Source: CAD feature listing. Evaluate the final solid. Frame: model axes, mm. A direction names the side the tool comes from. Round coordinates to 2 decimals unless told otherwise and drop trailing zeros. Order: outer loops, then holes, each group sorted by start corner. A loop starts at its lowest first (then second) coordinate and runs counter-clockwise, first axis right, second up. Notation, with made-up numbers: (68.25, -22) - (96.25, -22) arc R31 ccw to (96.25, 2) - close; hole circle Ø11 at (57, 14). An arc over 180 degrees is marked (long way). Return JSON: item names as keys, results as strings. Group by question number.
1) Section C-C, the plane y = 17.5. Return loops of the section in (x, z).
2) Ray query, line 1 (Y direction, x = 24.5, z = 0.05); line 2 (Y direction, x = 24.5, z = 9); line 3 (X direction, y = 18.5, z = 1). Return the intervals inside material, ascending. Write a range as from..to.
3) Section A-A, the plane x = -24.5. Return loops of the section in (y, z).
4) Section D-D, the plane x = 21.5. Return loops of the section in (y, z), plus the area to 4 significant figures.
5) Mould query, pull axis Y, two halves, no side actions, for faces 1 (the flat face through (28, 22.5, 5)), 2 (the flat face through (20, 18, 5)), 3 (the flat face through (27, 12.5, 5)). Classes: pulls with the +Y half, pulls with the -Y half, needs draft (parallel to the pull), parting line crosses it, or undercut.
6) Access query for faces 4 (the flat face through (35, 17, 5)), 5 (the flat face through (31, 18, 0.1)). Directions: +Z, -Z, +X, -X, +Y, -Y. A direction counts if a zero-diameter tool reaches every point of the face in a straight line with its end or side. Return the directions, or none.
7) Contact query for flat-ended pins moving along their axis: P1, Ø2.5, axis at x = 24.5, y = 24.5, coming from the -Z side; P2, Ø6.5, axis at x = -24.5, y = 24.5, coming from the +Z side; P3, Ø5, axis at y = 19, z = 7, coming from the -X side. Output: stop coordinate, or through.
Autodesk Inventor part; units mm, degrees
ref_plane "YZ Plane" through (0, 0, 0) normal (1, 0, 0) x (0, 1, 0)
ref_plane "XZ Plane" through (0, 0, 0) normal (0, 1, 0) x (-1, 0, 0)
ref_plane "XY Plane" through (0, 0, 0) normal (0, 0, 1) x (1, 0, 0)
sketch "스케치2" plane through (0, 0, 0) normal (0, 0, 1) x (1, 0, 0)
  line L0 (-27.5, 27.5) -> (27.5, 27.5)
  line L1 (27.5, 27.5) -> (27.5, -27.5)
  line L2 (27.5, -27.5) -> (-27.5, -27.5)
  line L3 (-27.5, -27.5) -> (-27.5, 27.5)
  line L4 (-27.5, 27.5) -> (27.5, -27.5) construction
  line L5 (27.5, 27.5) -> (-27.5, -27.5) construction
  point P0 (0, 0)
  dimension "d0" = 55
  dimension "d1" = 55
extrude "돌출1" add sketch "스케치2" along normal blind 0.1
sketch "스케치3" plane through (0, 0, 0.1) normal (0, 0, 1) x (1, 0, 0)
  line L0 (27.5, -27.5) -> (27.5, 27.5)
  line L1 (27.5, 27.5) -> (-27.5, 27.5)
  circle A0 centre (24.5, 24.5) radius 3
  circle A1 centre (-24.5, 24.5) radius 3
  circle A2 centre (-24.5, -24.5) radius 3
  circle A3 centre (24.5, -24.5) radius 3
  line L2 (-27.5, 27.5) -> (-27.5, -27.5)
  line L3 (-27.5, -27.5) -> (27.5, -27.5)
  circle A4 centre (24.5, 24.5) radius 2
  circle A5 centre (-24.5, 24.5) radius 2
  circle A6 centre (-24.5, -24.5) radius 2
  circle A7 centre (24.5, -24.5) radius 2
  point P0 (0, 0)
  dimension "d5" = 6
  dimension "d6" = 6
  dimension "d7" = 6
  dimension "d8" = 6
  dimension "d9" = 4
  dimension "d10" = 4
  dimension "d11" = 4
  dimension "d12" = 4
extrude "돌출2" cut sketch "스케치3" against normal up to surface (0.1 mm away) contours A4 | A5 | A6 | A7
sketch "스케치4" plane through (0, 0, 0.1) normal (0, 0, 1) x (1, 0, 0)
  line L0 (20, 12.5) -> (35, 12.5)
  line L1 (35, 12.5) -> (35, 22.5)
  line L2 (35, 22.5) -> (20, 22.5)
  line L3 (20, 22.5) -> (20, 12.5)
  line L4 (20, 12.5) -> (35, 22.5) construction
  line L5 (35, 12.5) -> (20, 22.5) construction
  line L6 (27.5, -27.5) -> (27.5, 27.5)
  circle A0 centre (24.5, 24.5) radius 2
  point P0 (0, 0)
  point P1 (27.5, 17.5)
  dimension "d15" = 15
  dimension "d16" = 10
extrude "돌출3" add sketch "스케치4" along normal blind 10 contours L3 L2 L6 L0 | L6 L2 L1 L0
properties part number "모터드라이버"
Geometry check:
{
 "1": {"outline": "(-27.5, 0) - (27.5, 0) - (27.5, 0.1) - (35, 0.1) - (35, 10.1) - (20, 10.1) - (20, 0.1) - (-27.5, 0.1) - close"},
 "2": {"line 1": "-27.5..-26.5, -22.5..22.5, 26.5..27.5", "line 2": "12.5..22.5", "line 3": "20..35"},
 "3": {"outline": "(-27.5, 0) - (-26.5, 0) - (-26.5, 0.1) - (-27.5, 0.1) - close; (-22.5, 0) - (22.5, 0) - (22.5, 0.1) - (-22.5, 0.1) - close; (26.5, 0) - (27.5, 0) - (27.5, 0.1) - (26.5, 0.1) - close"},
 "4": {"outline": "(-27.5, 0) - (27.5, 0) - (27.5, 0.1) - (22.5, 0.1) - (22.5, 10.1) - (12.5, 10.1) - (12.5, 0.1) - (-27.5, 0.1) - close", "area": "105.5 mm2"},
 "5": {"face 1": "pulls with the +Y half", "face 2": "needs draft", "face 3": "pulls with the -Y half"},
 "6": {"face 4": "+Z, -Z, +X, +Y, -Y", "face 5": "-Z, +X, +Y, -Y"},
 "7": {"P1": "through", "P2": "z = 0.1", "P3": "x = 20"}
}
